Check sheet for the drawn part. Datum: minimum x, y, z corner. Units: mm. A direction names the side the tool comes from. Round coordinates to 2 decimals unless told otherwise and drop trailing zeros. Write each loop counter-clockwise with the first axis right and the second up, starting at its lowest first coordinate (ties: lowest second). Pieces come first, ordered by that corner, then holes. Notation, with made-up numbers: (75, -39) - (120, -39) arc R34 ccw to (120, -5) - close; hole circle Ø4 at (50.25, 46). An arc over 180 degrees is marked (long way). Answer as a JSON object with one key per item and string values. Group by question number.
1) Section check D-D (x = 16.25). Enter the section's corners in (y, z), then the cut area to 3 significant figures.
2) Thickness scan on line 1 (Y direction, x = 6, z = 1.05); line 2 (Z direction, x = 16.95, y = 9); line 3 (Y direction, x = 3.75, z = 4.5). Record the ranges inside material, lowest first.
3) Go/stop test with flat-tipped pins: pin 1 Ø3 at (x, y) = (6, 6) entering from +Z; pin 2 Ø7.5 at (y, z) = (9, 7) entering from -X; pin 3 Ø7.5 at (x, y) = (6.5, 9.5) entering from +Z; pin 4 Ø4.5 at (x, z) = (8, 9) entering from +Y. Record where each tip stops, or that it passes through.
4) Mould release check, pull along X, two halves, no side actions. Record for the marked faces 3, 4, 5 and 6: +X half, -X half, draft (parallel to the pull), parting line (faces both ways), or undercut.
5) Section check B-B (x = 6). Enter the section's corners in (y, z).
6) Section check C-C (z = 1.5). Enter the section's corners in (x, y).
7) Set-up check for the marked faces 1 and 2: record each of +Z, -Z, +X, -X, +Y, -Y from which the full face is reachable in a straight line by a thin tool's end or side.
8) Section check A-A (y = 9). Enter the section's corners in (x, z).
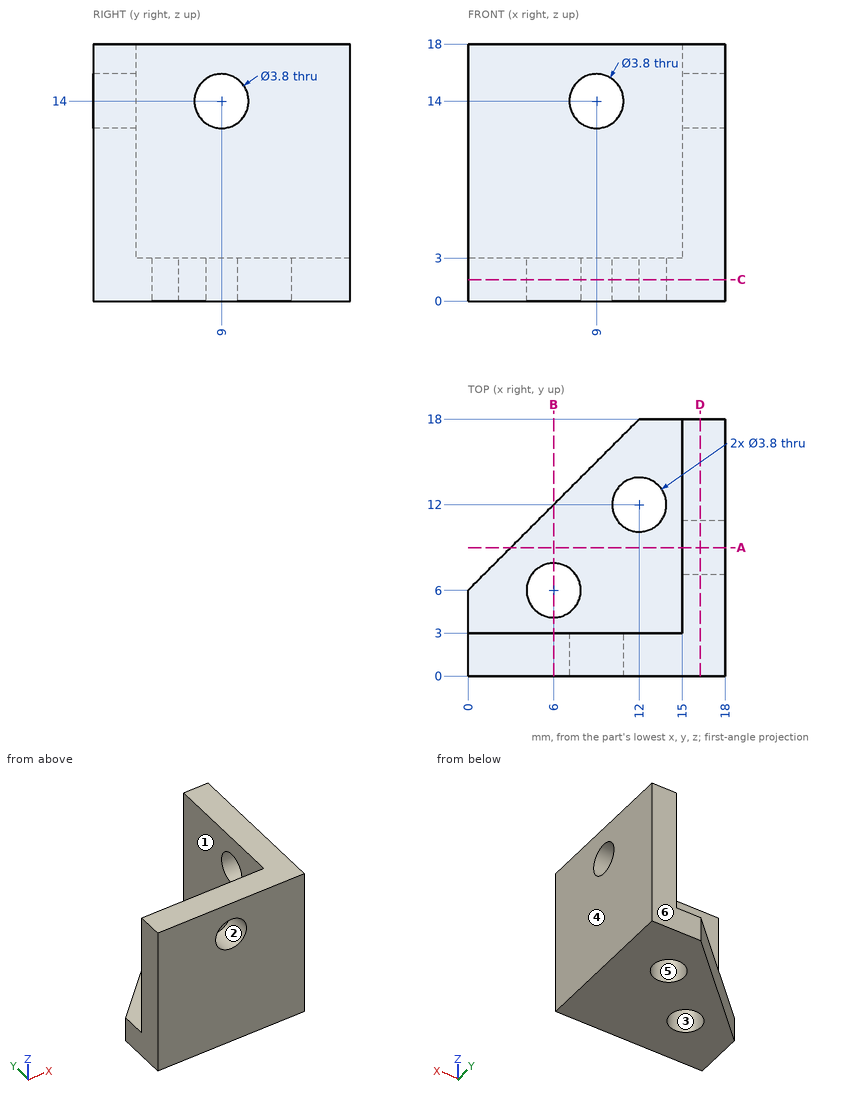
Returned:
{
 "1": {"outline": "(0, 0) - (18, 0) - (18, 18) - (0, 18) - close; hole circle Ø3.8 at (9, 14)", "area": "313 mm2"},
 "2": {"line 1": "0 to 4.1, 7.9 to 12", "line 2": "0 to 12.1, 15.9 to 18", "line 3": "0 to 3"},
 "3": {"pin 1": "through", "pin 2": "x = 15", "pin 3": "z = 3", "pin 4": "y = 3"},
 "4": {"face 3": "undercut", "face 4": "+X half", "face 5": "undercut", "face 6": "draft"},
 "5": {"outline": "(0, 0) - (4.1, 0) - (4.1, 3) - (3, 3) - (3, 18) - (0, 18) - close; (7.9, 0) - (12, 0) - (12, 3) - (7.9, 3) - close"},
 "6": {"outline": "(0, 0) - (18, 0) - (18, 18) - (12, 18) - (0, 6) - close; hole circle Ø3.8 at (6, 6); hole circle Ø3.8 at (12, 12)"},
 "7": {"face 1": "+Z, -X, +Y", "face 2": "+Y, -Y"},
 "8": {"outline": "(3, 0) - (18, 0) - (18, 12.1) - (15, 12.1) - (15, 3) - (3, 3) - close; (15, 15.9) - (18, 15.9) - (18, 18) - (15, 18) - close"}
}
